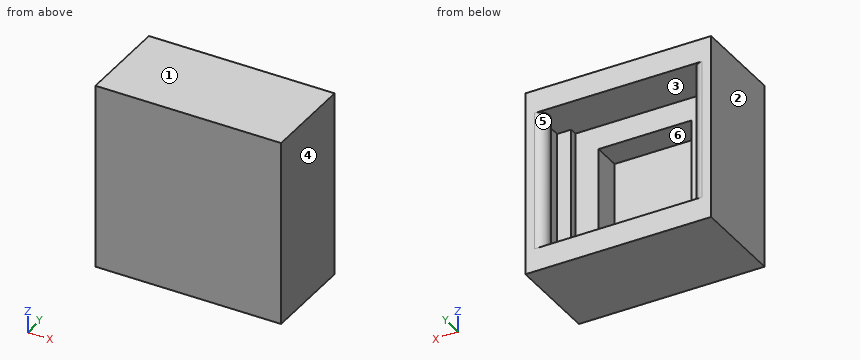
Autodesk Inventor part; units mm, degrees
ref_plane "Work Plane1" through (-25.4, 0, -12.7) normal (0, 0, 1) x (1, 0, 0)
ref_plane "Work Plane2" through (-12.7, 0, 0) normal (1, 0, 0) x (0, 0, -1)
ref_plane "YZ Plane" through (0, 0, 0) normal (1, 0, 0) x (0, 1, 0)
sketch "Sketch1" plane through (0, 0, 0) normal (0, 1, 0) x (-1, 0, 0)
  line L0 (0, 0) -> (25.4, 0)
  line L1 (25.4, 0) -> (25.4, -25.4)
  line L2 (25.4, -25.4) -> (0, -25.4)
  line L3 (0, -25.4) -> (0, 0)
  dimension "d0" = 25.4
  dimension "d1" = 25.4
extrude "Extrusion1" add sketch "Sketch1" along normal blind 12.7
shell "Shell1" thickness 6.35 removed faces 1 at (-8.4667, 12.7, -8.4667)
sketch "Sketch2" plane through (0, 12.7, 0) normal (0, 1, 0) x (1, 0, 0)
  line L0 (-22.225, 22.225) -> (-3.175, 22.225)
  line L1 (-3.175, 22.225) -> (-3.175, 3.175)
  line L2 (-3.175, 3.175) -> (-22.225, 3.175)
  line L3 (-22.225, 3.175) -> (-22.225, 22.225)
  line L4 (0, 0) -> (0, 25.4)
  line L5 (0, 25.4) -> (-25.4, 25.4)
  line L6 (-19.05, 19.05) -> (-6.35, 19.05)
  line L7 (-6.35, 19.05) -> (-6.35, 6.35)
  line L8 (-19.05, 19.05) -> (-6.35, 19.05)
  line L9 (-6.35, 19.05) -> (-6.35, 6.35)
  line L10 (-6.35, 6.35) -> (-19.05, 6.35)
  line L11 (-19.05, 6.35) -> (-19.05, 19.05)
  dimension "d5" = 19.05
  dimension "d6" = 19.05
  dimension "d7" = 3.175
  dimension "d8" = 3.175
extrude "Extrusion2" cut sketch "Sketch2" against normal blind 10.16 contours L6 L7 L10 L11
extrude "Extrusion3" cut sketch "Sketch2" against normal blind 6.35
ref_plane "Work Plane1" through (-25.4, 0, -12.7) normal (0, 0, 1) x (1, 0, 0)
ref_plane "Work Plane2" through (-12.7, 0, 0) normal (1, 0, 0) x (0, 0, -1)
sketch "Sketch3" plane through (-25.4, 0, -12.7) normal (0, 0, 1) x (1, 0, 0)
  line L0 (25.4, 12.7) -> (0, 12.7)
  circle A0 centre (1.27, 11.43) radius 1.27
  line L1 (0, 0) -> (0, 12.7)
  circle A1 centre (24.13, 11.43) radius 1.27
  line L2 (25.4, 0) -> (25.4, 12.7)
  line L3 (0, 12.7) -> (1.27, 12.7)
  line L4 (1.27, 12.7) -> (1.27, 7.366)
  line L5 (1.27, 7.366) -> (0, 7.366)
  line L6 (0, 7.366) -> (0, 12.7)
  line L7 (0, 12.7) -> (3.81, 12.7)
  line L8 (3.81, 12.7) -> (3.81, 7.366)
  line L9 (3.81, 7.366) -> (0, 7.366)
  line L10 (0, 7.366) -> (0, 12.7)
  line L11 (25.4, 0) -> (25.4, 12.7)
  line L12 (25.4, 12.7) -> (24.13, 12.7)
  line L13 (24.13, 12.7) -> (24.13, 7.366)
  line L14 (24.13, 7.366) -> (25.4, 7.366)
  line L15 (25.4, 7.366) -> (25.4, 12.7)
  line L16 (25.4, 12.7) -> (21.59, 12.7)
  line L17 (21.59, 12.7) -> (21.59, 7.366)
  line L18 (21.59, 7.366) -> (25.4, 7.366)
  line L19 (25.4, 7.366) -> (25.4, 12.7)
  point P0 (24.13, 10.16)
  point P1 (24.13, 12.7)
  point P2 (1.27, 7.366)
  point P3 (3.81, 12.7)
  point P4 (1.27, 12.7)
  point P5 (1.27, 10.16)
  dimension "d16" = 2.54
  dimension "d17" = 1.27
  dimension "d18" = 1.27
  dimension "d20" = 2.54
  dimension "d21" = 1.27
  dimension "d22" = 1.27
  dimension "d23" = 1.27
  dimension "d24" = 5.334
  dimension "d25" = 1.27
  dimension "d26" = 5.334
  dimension "d27" = 3.81
  dimension "d28" = 5.334
  dimension "d29" = 5.334
  dimension "d30" = 3.81
extrude "Extrusion4" cut sketch "Sketch3" along normal mid plane 19.05 contours L8 L9 L4 A0 L0 | A1 L13 L18 L17 L0
sketch "Sketch4" plane through (-12.7, 0, 0) normal (1, 0, 0) x (0, 0, -1)
  circle A0 centre (1.27, 11.43) radius 1.27
  circle A1 centre (24.13, 11.43) radius 1.27
  line L0 (0, 12.7) -> (25.4, 12.7)
  line L1 (25.4, 0) -> (25.4, 12.7)
  line L2 (0, 0) -> (0, 12.7)
  line L3 (0, 12.7) -> (1.27, 12.7)
  line L4 (1.27, 12.7) -> (1.27, 8.89)
  line L5 (1.27, 8.89) -> (0, 8.89)
  line L6 (0, 8.89) -> (0, 12.7)
  line L7 (25.4, 12.7) -> (24.13, 12.7)
  line L8 (24.13, 12.7) -> (24.13, 8.89)
  line L9 (24.13, 8.89) -> (25.4, 8.89)
  line L10 (25.4, 8.89) -> (25.4, 12.7)
  line L11 (0, 12.7) -> (3.81, 12.7)
  line L12 (3.81, 12.7) -> (3.81, 8.89)
  line L13 (3.81, 8.89) -> (0, 8.89)
  line L14 (0, 8.89) -> (0, 12.7)
  line L15 (25.4, 12.7) -> (21.59, 12.7)
  line L16 (21.59, 12.7) -> (21.59, 8.89)
  line L17 (21.59, 8.89) -> (25.4, 8.89)
  line L18 (25.4, 8.89) -> (25.4, 12.7)
  dimension "d33" = 2.54
  dimension "d34" = 2.54
  dimension "d35" = 1.27
  dimension "d36" = 1.27
  dimension "d37" = 1.27
  dimension "d38" = 1.27
  dimension "d39" = 1.27
  dimension "d40" = 3.81
  dimension "d41" = 1.27
  dimension "d42" = 3.81
  dimension "d43" = 3.81
  dimension "d44" = 3.81
  dimension "d45" = 3.81
  dimension "d46" = 3.81
properties part number "boxtest"
Verification items for the finished model (mm, model axes). Face numbers are marked on the shaded views. A direction names the side the tool comes from. Round coordinates to 2 decimals unless told otherwise and drop trailing zeros. Order: outer loops, then holes, each group sorted by start corner. A loop starts at its lowest first (then second) coordinate and runs counter-clockwise, first axis right, second up.
1. Section check D-D on y = 11.43. Record the cut outline in (x, z) (3 decimals).
Final values:
outline: (-25.4, -25.4) - (0, -25.4) - (0, 0) - (-25.4, 0) - close; hole (-22.86, -22.225) - (-2.54, -22.225) - (-2.54, -3.175) - (-22.86, -3.175) - close
2. Section check A-A on y = 8.5. Record the cut outline in (x, z) (3 decimals).
Final values:
outline: (-25.4, -25.4) - (0, -25.4) - (0, 0) - (-25.4, 0) - close; hole (-24.13, -22.225) - (-1.27, -22.225) - (-1.27, -3.175) - (-24.13, -3.175) - close
3. Section check B-B on z = -12.25. Record the cut outline in (x, y) (3 decimals).
Final values:
outline: (-25.4, 0) - (0, 0) - (0, 12.7) - (-1.27, 12.7) arc R1.27 ccw to (-1.27, 10.16) - (-1.27, 7.366) - (-3.175, 7.366) - (-3.175, 6.35) - (-6.35, 6.35) - (-6.35, 2.54) - (-19.05, 2.54) - (-19.05, 6.35) - (-22.225, 6.35) - (-22.225, 7.366) - (-24.13, 7.366) - (-24.13, 10.16) arc R1.27 ccw to (-24.13, 12.7) - (-25.4, 12.7) - close
4. Thickness scan on L1, parallel to Z at x = -9.75, y = 9 (3 decimals); L2, parallel to X at y = 11.5, z = -21.75; L3, parallel to X at y = 8.25, z = -16.25. Record the ranges inside material, lowest first.
Final values:
L1: z = -25.4 to -22.225, -3.175 to 0
L2: x = -25.4 to -22.86, -2.54 to 0
L3: x = -25.4 to -24.13, -1.27 to 0
5. Access from +Z, -Z, +X, -X, +Y, -Y to the whole of each face (thin tool, end or side, straight path). Record for the marked faces 4, 5 and 6.
Final values:
face 4: +Z, -Z, +X, +Y, -Y
face 5: none
face 6: +Y
6. Release check for a two-part mould opening along X. For the marked faces 1, 2 and 3 record: +X half, -X half, draft (parallel to the pull), parting line (faces both ways), or undercut.
Final values:
face 1: draft
face 2: -X half
face 3: undercut
7. Go/stop test with flat-tipped pins: P1, Ø1, axis at x = -2.5, z = -9, coming from the +Y side; P2, Ø4, axis at x = -12, z = -13.5, coming from the +Y side. Record where each tip stops, or that it passes through.
Final values:
P1: stops at y = 12.47
P2: stops at y = 2.54
8. Section check C-C on x = -10. Record the cut outline in (y, z) (3 decimals), then the cut area to 3 significant figures.
Final values:
outline: (0, -25.4) - (12.7, -25.4) - (12.7, -22.225) - (6.35, -22.225) - (6.35, -19.05) - (2.54, -19.05) - (2.54, -6.35) - (6.35, -6.35) - (6.35, -3.175) - (12.7, -3.175) - (12.7, 0) - (0, 0) - close
area: 153 mm2
